Geometry: final body of the model. Coordinates: model frame, mm. A direction names the side the tool comes from. Give positions to 0.01 mm unless a question says otherwise; leave off trailing zeros. Order: outer loops, then holes, each group sorted by start corner. A loop starts at its lowest first (then second) coordinate and runs counter-clockwise, first axis right, second up. Notation, with made-up numbers: (43.5, 68.25) - (65.5, 68.25) arc R17 ccw to (65.5, 85.25) - close; hole circle Ø9 at (47, -23). An arc over 180 degrees is marked (long way). Use one line per item in the form item = value.
from build123d import *

# Parameters (mm, degrees)
SKETCH1_R           = 72.175
SKETCH1_R_2         = 20
BOSS_EXTRUDE1_DEPTH = 7.5
SKETCH3_R           = 30.5
CUT_EXTRUDE1_DEPTH  = 4
SKETCH4_R           = 2.5
CUT_EXTRUDE2_DEPTH  = 104.167151991


with BuildPart() as part:
    # Sketch1 → Boss-Extrude1 (new, symmetric)
    with BuildSketch(Plane(origin=(0, 0, 0), x_dir=(1, 0, 0), z_dir=(0, 1, 0))):
        with Locations(Location((0, 0, 0), (0, 0, 270))):
            Circle(SKETCH1_R)
        with Locations(Location((0, 0, 0), (0, 0, 270))):
            Circle(SKETCH1_R_2, mode=Mode.SUBTRACT)
    extrude(amount=BOSS_EXTRUDE1_DEPTH, both=True)

    # Sketch2 → Cut-Revolve1 (revolve, cut)
    with BuildSketch(Plane.XY, mode=Mode.PRIVATE) as cut_revolve1_sk:
        Polygon((72.175, -5.115), (72.175, 5.115), (70, 2.94), (70, -2.94), align=None)
    revolve(cut_revolve1_sk.sketch.rotate(Axis((0, 6.6, 0), (0, -1, 0)), 90), axis=Axis((0, 6.6, 0), (0, -1, 0)), mode=Mode.SUBTRACT)

    # Sketch3 → Cut-Extrude1 (cut)
    with BuildSketch(Plane.XZ.offset(7.5)):
        with Locations(Location((0, 0, 0), (0, 0, 270))):
            Circle(SKETCH3_R)
    extrude(amount=-CUT_EXTRUDE1_DEPTH, mode=Mode.SUBTRACT)

    # Sketch4 → Cut-Extrude2 (cut, through all)
    with BuildSketch(Plane(origin=(0, 7.5, 0), x_dir=(1, 0, 0), z_dir=(0, 1, 0))):
        with Locations(Location((62.5, 0, 0), (0, 0, 270))):
            Circle(SKETCH4_R)
        with Locations(Location((45, 31.622776602, 0), (0, 0, 270))):
            Circle(SKETCH4_R)
        with Locations(Location((45, -31.622776602, 0), (0, 0, 270))):
            Circle(SKETCH4_R)
    cut_extrude2 = extrude(amount=-CUT_EXTRUDE2_DEPTH, mode=Mode.SUBTRACT)

    # Mirror1: Cut-Extrude2 across plane
    add(cut_extrude2.mirror(Plane(origin=(0, 0, 0), x_dir=(0, 0, 1), z_dir=(1, 0, 0))), mode=Mode.SUBTRACT)


solid = part.part
(1) Reachability of faces 4 (the face through (-43.917, 6.324, -57.276)), 5 (the face through (68.335, -0.041, -15.175)), 6 (the face through (-29.775, -5.528, 6.612)) from +Z, -Z, +X, -X, +Y, -Y: full face, straight path, thin tool, end or side. Return the list, or none.
Computed values:
face_4 = +Y, -Y
face_5 = none
face_6 = -Y
(2) Pull-direction query (Y, two-part tool) for faces 1 (the face through (43.48, 0.11, -33.61)), 2 (the face through (68.44, 3.05, -15.2)), 3 (the face through (1, -7.5, 31)); classes: released by +Y, released by -Y, zero draft, split by the parting line, or undercut.
Computed values:
face_1 = zero draft
face_2 = undercut
face_3 = released by -Y
(3) Cut plane A-A on z = 0. Output: boundary loops of the cut face in (x, y) (3 decimals), plus the area to 3 significant figures.
Computed values:
outline = (-72.175, -7.5) - (-65, -7.5) - (-65, 7.5) - (-72.175, 7.5) - (-72.175, 5.115) - (-70, 2.94) - (-70, -2.94) - (-72.175, -5.115) - close; (-60, -7.5) - (-30.5, -7.5) - (-30.5, -3.5) - (-20, -3.5) - (-20, 7.5) - (-60, 7.5) - close; (20, -3.5) - (30.5, -3.5) - (30.5, -7.5) - (60, -7.5) - (60, 7.5) - (20, 7.5) - close; (65, -7.5) - (72.175, -7.5) - (72.175, -5.115) - (70, -2.94) - (70, 2.94) - (72.175, 5.115) - (72.175, 7.5) - (65, 7.5) - close
area = 1,300 mm²
(4) Ray query, line 1 along X through (y, z) = (-1.5, 0); line 2 along Z through (x, y) = (-45, 3.75); line 3 along Z through (x, y) = (-43, 1.5). Return the intervals inside material, ascending.
Computed values:
line_1 = -70 to -65, -60 to -20, 20 to 60, 65 to 70
line_2 = -54.67 to -34.12, -29.12 to 29.12, 34.12 to 54.67
line_3 = -55.24 to -33.12, -30.12 to 30.12, 33.12 to 55.24
(5) Contact query for flat-ended pins moving along their axis: pin 1 Ø8 at (x, z) = (-45, 31.62) entering from -Y; pin 2 Ø4 at (y, z) = (-0.5, 36.5) entering from -X; pin 3 Ø4 at (y, z) = (-4.5, 3.5) entering from -X; pin 4 Ø4 at (y, z) = (5.5, -55.5) entering from -X. Output: stop coordinate, or through.
Computed values:
pin_1 = -7.5
pin_2 = -60.91
pin_3 = -72.16
pin_4 = -48.45
(6) Cut plane C-C on x = -45. Give the number of separate pieces and of enclosed holes in the cut face, plus the area to 3 significant figures.
Computed values:
separate_pieces = 3
enclosed_holes = 0
area = 1,500 mm²
(7) Cut plane B-B on x = 0. Output: boundary loops of the cut face in (y, z) (3 decimals).
Computed values:
outline = (-7.5, -72.175) - (-5.115, -72.175) - (-2.94, -70) - (2.94, -70) - (5.115, -72.175) - (7.5, -72.175) - (7.5, -20) - (-3.5, -20) - (-3.5, -30.5) - (-7.5, -30.5) - close; (-7.5, 30.5) - (-3.5, 30.5) - (-3.5, 20) - (7.5, 20) - (7.5, 72.175) - (5.115, 72.175) - (2.94, 70) - (-2.94, 70) - (-5.115, 72.175) - (-7.5, 72.175) - close
